Can you work these out from the model? Positions are in its coordinate system, mm. Face numbers are marked on the shaded views. A direction names the side the tool comes from. Round coordinates to 2 decimals unless told otherwise and drop trailing zeros. Loops run counter-clockwise (first coordinate to the right, second up) from the corner with the lowest first, then second, coordinate; pieces in that order, holes last. Notation, with made-up numbers: M 81.5,25.5 L 104.5,25.5 A31 ccw 104.5,59.5 Z; hole C -1.75,23.25 d11. An arc over 180 degrees is marked long. Return JSON: item names as keys, results as strings.
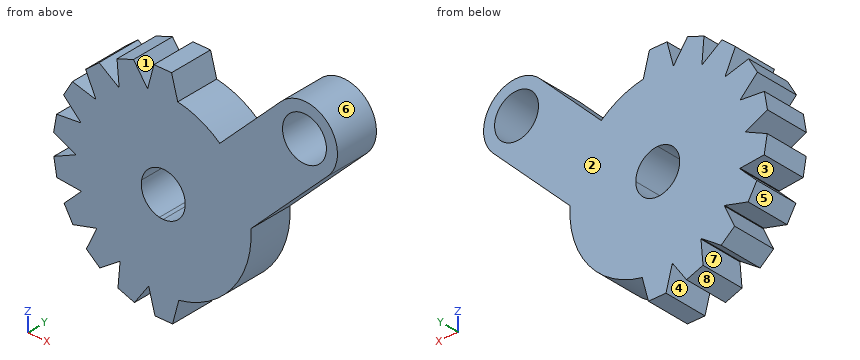
```python
from build123d import *

# Parameters (mm, degrees)
SALIENTE_EXTRUIR1_DEPTH = 10
MATRIZC1_COUNT          = 10
MATRIZC1_ANGLE          = 180
SALIENTE_EXTRUIR5_START = -10
CROQUIS2_R              = 5
SALIENTE_EXTRUIR5_DEPTH = 10


with BuildPart() as part:
    # Croquis1 → Saliente-Extruir1 (new body)
    with BuildSketch(Plane(origin=(0, 0, 0), x_dir=(1, 0, 0), z_dir=(0, 1, 0))):
        with BuildLine():
            Line((0, 5), (0, 20))
            Line((0, 20), (0, 24.969733164))
            Line((0, 24.969733164), (-1.883440248, 24.969733164))
            Line((-1.883440248, 24.969733164), (-3.287991504, 19.727876517))
            ThreePointArc((-3.287991504, 19.727876517), (-19.931853029, -1.649616571), (0, -20))
            Line((0, -20), (0, -5))
            ThreePointArc((0, -5), (-5, 0), (0, 5))
        make_face()
        with BuildLine():
            Line((0, 24.969733164), (0, 20))
            Line((0, 20), (0, 5))
            ThreePointArc((0, 5), (3.535533906, 3.535533906), (5, 0))
            ThreePointArc((5, 0), (3.535533906, -3.535533906), (0, -5))
            Line((0, -5), (0, -20))
            ThreePointArc((0, -20), (19.921238429, -1.773205983), (3.532445918, 19.685574054))
            Line((3.532445918, 19.685574054), (2.116559752, 24.969733164))
            Line((2.116559752, 24.969733164), (0, 24.969733164))
        make_face()
    saliente_extruir1 = extrude(amount=SALIENTE_EXTRUIR1_DEPTH)

    # MatrizC1: Saliente-Extruir1 ×10 about axis
    matrizc1_axis = Axis((0, 0, 0), (0, 1, 0))
    for i in range(1, MATRIZC1_COUNT):
        add(saliente_extruir1.rotate(matrizc1_axis, i * MATRIZC1_ANGLE / (MATRIZC1_COUNT - 1)))

    # Croquis2 → Saliente-Extruir5 (add)
    with BuildSketch(Plane.XZ.offset(SALIENTE_EXTRUIR5_START)):
        with BuildLine():
            Line((26.827116941, 29.295976121), (12.853727975, 15.322587155))
            ThreePointArc((12.853727975, 15.322587155), (17.859540741, 9.002044462), (19.962846781, 1.218502525))
            Line((19.962846781, 1.218502525), (37.433718659, 18.689374403))
            ThreePointArc((37.433718659, 18.689374403), (37.433718659, 29.295976121), (26.827116941, 29.295976121))
        make_face()
        with Locations(Location((32.1304178, 23.992675262, 0), (0, 0, 270))):
            Circle(CROQUIS2_R, mode=Mode.SUBTRACT)
    extrude(amount=SALIENTE_EXTRUIR5_DEPTH)


solid = part.part
```
Q1. On a 3-axis mill with a long thin cutter (end or side, diameter ignored), from which of +Z, -Z, +X, -X, +Y, -Y can I reach the whole of each face in a straight line? I mean the marked faces 1, 2, 3, 4 and 5. Say none if no direction works.
Results:
{"face 1": "+Z, +Y, -Y", "face 2": "+Z, -Z, +X, -X, +Y", "face 3": "-X, +Y, -Y", "face 4": "-Z, +Y, -Y", "face 5": "-Z, -X, +Y, -Y"}
Q2. If I drill on line 1 along Z through (x, y) = (31, 5.5); line 2 along Z through (x, y) = (28, 8.5); line 3 along X through (y, z) = (9.5, -21.5), over which ranges is the centre line in solid material (lowest first)?
Results:
{"line 1": "z = 12.26 to 19.12, 28.86 to 31.41", "line 2": "z = 9.26 to 21.17, 26.81 to 30.25", "line 3": "x = -10.19 to -4.67, -2.81 to 3.05"}
Q3. Thinking about a two-plate mould opening in X: for the marked faces 6, 7 and 8, which applies, pulls with the +X half, pulls with the -X half, needs draft (parallel to the pull), parting line crosses it, or undercut?
Results:
{"face 6": "parting line crosses it", "face 7": "undercut", "face 8": "pulls with the -X half"}
Q4. Suppose I cut it at B-B, the plane z = -16. Please give me the cut outline in (x, y).
Results:
{"outline": "M -16.6,0 L 12,0 L 12,10 L -16.6,10 Z"}
Q5. Suppose I cut it at A-A, the plane x = 34. Please give me the cut outline in (y, z).
Results:
{"outline": "M 0,15.26 L 10,15.26 L 10,19.36 L 0,19.36 Z; M 0,28.63 L 10,28.63 L 10,31.26 L 0,31.26 Z"}
Q6. Suppose I cut it at D-D, the plane x = 16. Please give me the cut outline in (y, z).
Results:
{"outline": "M 0,-12 L 10,-12 L 10,18.47 L 0,18.47 Z"}
Q7. Suppose I cut it at C-C, the plane y = 4.5. State how many separate pieces and enclosed holes the cut face has, plus the area to 3 significant figures.
Results:
{"separate pieces": "1", "enclosed holes": "2", "area": "1,780 mm2"}
Q8. I'm going to push flat-ended pins straight in: pin 1 Ø4 at (x, y) = (-8.5, 8) entering from +Z; pin 2 Ø1.2 at (x, y) = (0.5, 2.5) entering from +Z; pin 3 Ø3 at (y, z) = (7.5, -17.5) entering from +X. Where does each tip first touch, or does it pass through?
Results:
{"pin 1": "stops at z = 24.11", "pin 2": "stops at z = 24.97", "pin 3": "stops at x = 12"}
